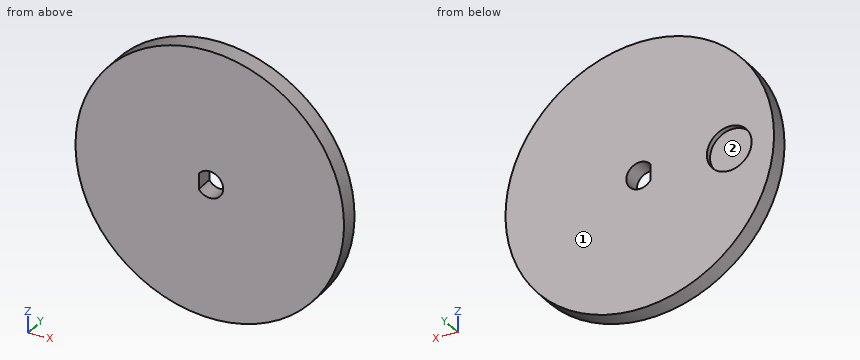
```python
from build123d import *

# Parameters (mm, degrees)
SKETCH1_R           = 30
BOSS_EXTRUDE1_DEPTH = 4
SKETCH2_R           = 5
CUT_EXTRUDE1_DEPTH  = 1.2


with BuildPart() as part:
    # Sketch1 → Boss-Extrude1 (new body)
    with BuildSketch(Plane(origin=(0, 0, 0), x_dir=(1, 0, 0), z_dir=(0, 1, 0))):
        with Locations(Location((0, 0, 0), (0, 0, 270))):
            Circle(SKETCH1_R)
        with BuildLine():
            Line((-2.45, 1.731328969), (-2.45, 0))
            Line((-2.45, 0), (-2.45, -1.731328969))
            ThreePointArc((-2.45, -1.731328969), (3, 0), (-2.45, 1.731328969))
        make_face(mode=Mode.SUBTRACT)
    extrude(amount=BOSS_EXTRUDE1_DEPTH)

    # Sketch2 → Cut-Extrude1 (cut)
    with BuildSketch(Plane(origin=(0, 4, 0), x_dir=(1, 0, 0), z_dir=(0, 1, 0))):
        with Locations(Location((-20, 0, 0), (0, 0, 270))):
            Circle(SKETCH2_R)
    extrude(amount=-CUT_EXTRUDE1_DEPTH, mode=Mode.SUBTRACT)


solid = part.part
```
Here's how the part is built. I have some questions about the finished solid (model axes, mm). Face numbers are marked on the shaded views. Coordinates: 2 decimals unless noted, no trailing zeros. Order: outer loops, then holes, each group sorted by start corner. A loop starts at its lowest first (then second) coordinate and runs counter-clockwise, first axis right, second up. Notation, with made-up numbers: M 9.5,13.25 L 27.5,13.25 A20 ccw 27.5,19.25 Z; hole C -16.75,-10.75 d6. An arc over 180 degrees is marked long. Answer as a JSON object with one key per item and string values. Group by question number.
(1) If we mould it in two halves opening along Z, with no side actions, what happens to the marked faces 1 and 2? For each: released by +Z, released by -Z, zero draft, split by the parting line, or undercut.
(2) Suppose I cut it at A-A, the plane x = 0. Please give me the cut outline in (y, z).
(3) Suppose I cut it at B-B, the plane z = 0. Please give me the cut outline in (x, y).
(4) Suppose I cut it at D-D, the plane x = -21. Please give me the cut outline in (y, z), then the cut area to 3 significant figures.
(5) For pin 1 (9 mm diameter, centred on x = -20, z = 0, fed in from +Y), with a flat end and sliding along its axis, tell me the tip position at first contact or that it passes through.
(6) I need wall thicknesses on probe 1 along X at (y, z) = (3.7, 0); probe 2 along Z at (x, y) = (-23, 3); probe 3 along Z at (x, y) = (-2, 2.7). Which ranges of each line are inside material? Lowest first, please.
(7) Suppose I cut it at C-C, the plane y = 1.4. Please give me the cut outline in (x, z), then the cut area to 3 significant figures.
Values found:
{
 "1": {"face 1": "zero draft", "face 2": "undercut"},
 "2": {"outline": "M 0,-30 L 4,-30 L 4,-3 L 0,-3 Z; M 0,3 L 4,3 L 4,30 L 0,30 Z"},
 "3": {"outline": "M -30,0 L -2.45,0 L -2.45,4 L -15,4 L -15,2.8 L -25,2.8 L -25,4 L -30,4 Z; M 3,0 L 30,0 L 30,4 L 3,4 Z"},
 "4": {"outline": "M 0,-21.42 L 4,-21.42 L 4,-4.9 L 2.8,-4.9 L 2.8,4.9 L 4,4.9 L 4,21.42 L 0,21.42 Z", "area": "160 mm^2"},
 "5": {"pin 1": "stops at y = 2.8"},
 "6": {"probe 1": "x = -30 to -25, -15 to -2.45, 3 to 30", "probe 2": "z = -19.26 to -4, 4 to 19.26", "probe 3": "z = -29.93 to -2.24, 2.24 to 29.93"},
 "7": {"outline": "C 0,0 d60; hole M -2.45,-1.73 A3 ccw long -2.45,1.73 Z", "area": "2,800 mm^2"}
}
